Read the model definition and answer for the solid it produces. Units are mm, in the model's axes. Face numbers are marked on the shaded views. A direction names the side the tool comes from. Coordinates: 2 decimals unless noted, no trailing zeros. Write each loop counter-clockwise with the first axis right and the second up, starting at its lowest first coordinate (ties: lowest second). Pieces come first, ordered by that corner, then holes. Notation, with made-up numbers: (-7, 51) -> (41, 51) arc R38 ccw to (41, 89) -> close; hole circle Ø8 at (12, -35). An arc over 180 degrees is marked (long way). One line per item, written item: value. Start each with the question number.
1. For a pull along Y with two mould halves and no side action, classify the marked faces 4, 5, 6 and 7 as pulls with the +Y half, pulls with the -Y half, needs draft (parallel to the pull), parting line crosses it, or undercut.
2. Find section C-C, the plane z = 2.5. Write down the section's boundary in (x, y).
3. Find section A-A, the plane x = -20. Write down the section's boundary in (y, z).
4. For the marked faces 1, 2 and 3, determine the directions among +Z, -Z, +X, -X, +Y, -Y from which every point of the face is accessible in a straight line to the end or side of a thin tool.
5. Given P1, Ø4, axis at x = -15.5, y = 69, coming from the +Z side; P2, Ø4, axis at x = -5.5, z = 12.5, coming from the +Y side, each flat-ended and moving along its own axis, determine where each tip first touches the part or whether it passes through.
6. Consider line 1 along X through (y, z) = (34, 3); line 2 along Y through (x, z) = (-20, 11.5); line 3 along Y through (x, z) = (-8, 8.25). Determine where each line is inside the solid, lowest interval first.
7. Find section D-D, the plane x = -3. Write down the section's boundary in (y, z), and give its area (3 significant figures).
8. Find section B-B, the plane y = 20. Write down the section's boundary in (x, z).
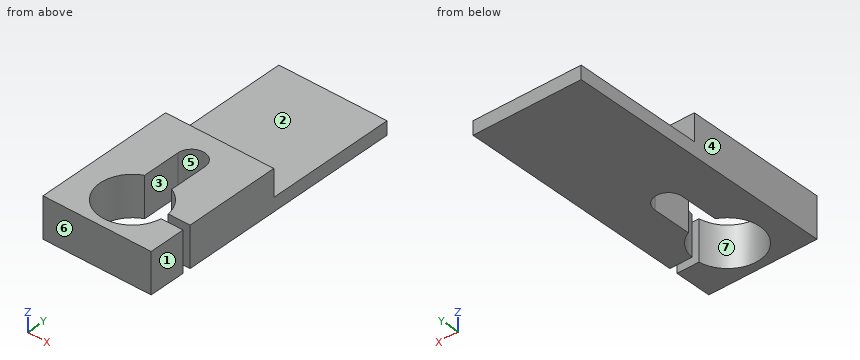
```python
from build123d import *

# Parameters (mm, degrees)
EXTRUSION1_DEPTH = 15
ESQUISSE2_W      = 40
ESQUISSE2_H      = 48
EXTRUSION2_DEPTH = 10


with BuildPart() as part:
    # Esquisse1 → Extrusion1 (new body)
    with BuildSketch(Plane.XY):
        with BuildLine():
            Line((0, 0), (-40, 0))
            Line((-40, 0), (-40, 100))
            Line((-40, 100), (0, 100))
            Line((0, 100), (0, 16.5))
            Line((0, 16.5), (-8.0941191, 16.5))
            ThreePointArc((-8.0941191, 16.5), (-10.32616063, 22.100481099), (-15, 25.908712115))
            Line((-15, 25.908712115), (-15, 40))
            ThreePointArc((-15, 40), (-20, 45), (-25, 40))
            Line((-25, 40), (-25, 25.908712115))
            ThreePointArc((-25, 25.908712115), (-27.100481099, 5.32616063), (-8.0941191, 13.5))
            Line((-8.0941191, 13.5), (0, 13.5))
            Line((0, 13.5), (0, 0))
        make_face()
    extrude(amount=EXTRUSION1_DEPTH)

    # Esquisse2 → Extrusion2 (cut)
    with BuildSketch(Plane.XY.offset(15)):
        with Locations((-20, 76)):
            Rectangle(ESQUISSE2_W, ESQUISSE2_H)
    extrude(amount=-EXTRUSION2_DEPTH, mode=Mode.SUBTRACT)


solid = part.part
```
Answer block:
1. face 4: needs draft
1. face 5: undercut
1. face 6: pulls with the -Y half
1. face 7: undercut
2. outline: (-40, 0) -> (0, 0) -> (0, 13.5) -> (-8.09, 13.5) arc R12 cw (long way) to (-25, 25.91) -> (-25, 40) arc R5 cw to (-15, 40) -> (-15, 25.91) arc R12 cw to (-8.09, 16.5) -> (0, 16.5) -> (0, 100) -> (-40, 100) -> close
3. outline: (0, 0) -> (3, 0) -> (3, 15) -> (0, 15) -> close; (45, 0) -> (100, 0) -> (100, 5) -> (52, 5) -> (52, 15) -> (45, 15) -> close
4. face 1: +Z, -Z, +X, +Y, -Y
4. face 2: +Z, +X, -X, +Y
4. face 3: +Z, -Z
5. P1: stops at z = 5
5. P2: stops at y = 52
6. line 1: x = -40 to -25, -15 to 0
6. line 2: y = 0 to 3, 45 to 52
6. line 3: y = 0 to 13.5, 16.5 to 52
7. outline: (0, 0) -> (13.5, 0) -> (13.5, 15) -> (0, 15) -> close; (16.5, 0) -> (100, 0) -> (100, 5) -> (52, 5) -> (52, 15) -> (16.5, 15) -> close
7. area: 975 mm2
8. outline: (-40, 0) -> (-30.91, 0) -> (-30.91, 15) -> (-40, 15) -> close; (-9.09, 0) -> (0, 0) -> (0, 15) -> (-9.09, 15) -> close
